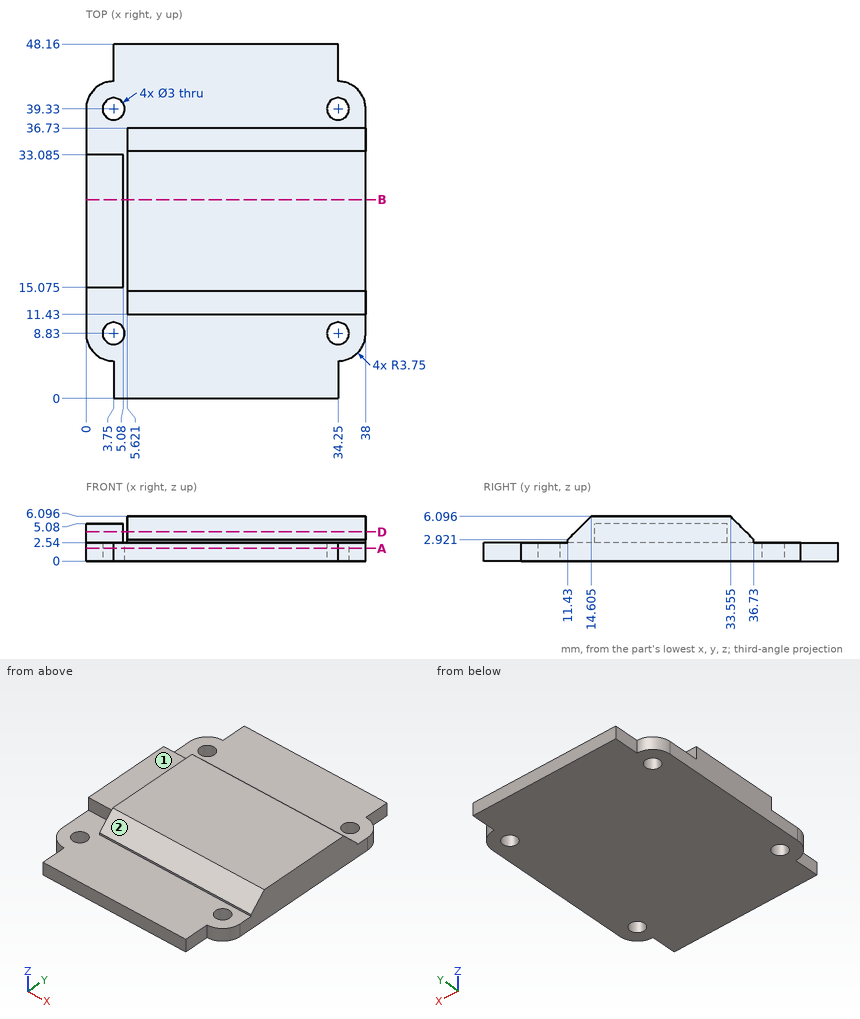
For this review, use the dimensioned drawing (mm, ordinates from the lowest corner) and the shaded views. A direction names the side the tool comes from. Give positions to 0.01 mm unless a question says otherwise; leave off trailing zeros. Order: outer loops, then holes, each group sorted by start corner. A loop starts at its lowest first (then second) coordinate and runs counter-clockwise, first axis right, second up. Notation, with made-up numbers: M 45,34.25 L 95,34.25 A20 cw 95,54.25 Z; hole C -38,56 d6. An arc over 180 degrees is marked long. One line per question, with ' | ' between items. Start each with the question number.
1) Clearance check with flat-ended pins moving along their axes: P1, Ø4, axis at x = 3.75, y = 39.33, coming from the +Z side; P2, Ø5, axis at x = 26, y = 40, coming from the -Z side; P3, Ø1.3, axis at y = 44.5, z = 1.5, coming from the -X side; P4, Ø2, axis at y = 47, z = 1, coming from the +X side. State where each tip first meets the part, or that it passes through.
2) Consider section A-A, the plane z = 1.75. Give the boundary of the cut face in (x, y), then the cut area to 3 significant figures.
3) Wall thickness on L1, parallel to Z at x = 33, y = 46; L2, parallel to X at y = 28, z = 3.25; L3, parallel to Z at x = 4, y = 20: over which ranges is each line inside the solid? List them lowest first. Write a range as from..to.
4) For the marked faces 1 and 2, list the 3-axis set-ups (+Z, -Z, +X, -X, +Y, -Y) from which the entire face can be reached by the end or side of a thin tool; tool diameter is ignored.
5) Consider section D-D, the plane z = 4. Give the boundary of the cut face in (x, y) (1 decimal).
6) Consider section B-B, the plane y = 27. Give the boundary of the cut face in (x, z).
Found:
1) P1: stops at z = 2.54 | P2: stops at z = 0 | P3: stops at x = 3.75 | P4: stops at x = 34.25
2) outline: M 0,8.83 A3.75 ccw 3.75,5.08 L 3.75,0 L 34.25,0 L 34.25,5.08 A3.75 ccw 38,8.83 L 38,39.33 A3.75 ccw 34.25,43.08 L 34.25,48.16 L 3.75,48.16 L 3.75,43.08 A3.75 ccw 0,39.33 Z; hole C 3.75,8.83 d3; hole C 3.75,39.33 d3; hole C 34.25,8.83 d3; hole C 34.25,39.33 d3 | area: 1,710 mm²
3) L1: z = 0..2.54 | L2: x = 0..5.08, 5.62..38 | L3: z = 0..5.08
4) face 1: +Z, -X, +Y, -Y | face 2: +Z, +X, -X, -Y
5) outline: M 0,15.1 L 5.1,15.1 L 5.1,33.1 L 0,33.1 Z; M 5.6,12.5 L 38,12.5 L 38,35.7 L 5.6,35.7 Z
6) outline: M 0,0 L 38,0 L 38,6.1 L 5.62,6.1 L 5.62,2.54 L 5.08,2.54 L 5.08,5.08 L 0,5.08 Z
